from build123d import *

# Parameters (mm, degrees)
PAD_DEPTH    = 9
SKETCH001_R  = 2.5
POCKET_DEPTH = 10


with BuildPart() as part:
    # Sketch → Pad (new body)
    with BuildSketch(Plane.YZ):
        with BuildLine():
            Line((-3.5, 0), (-3.403323, 1.122173))
            ThreePointArc((-3.31749, 2.118482), (-3.858561, 1.663244), (-3.403323, 1.122173))
            Line((-3.31749, 2.118482), (-3.220813, 3.240655))
            ThreePointArc((-3.13498, 4.236964), (-3.676052, 3.781726), (-3.220813, 3.240655))
            Line((-3.13498, 4.236964), (-3.038304, 5.359137))
            ThreePointArc((-2.95247, 6.355446), (-3.493542, 5.900208), (-3.038304, 5.359137))
            Line((-2.95247, 6.355446), (-2.855794, 7.477619))
            ThreePointArc((-2.76996, 8.473929), (-3.311032, 8.01869), (-2.855794, 7.477619))
            Line((-2.76996, 8.473929), (-2.673284, 9.596101))
            ThreePointArc((-2.58745, 10.592411), (-3.128522, 10.137173), (-2.673284, 9.596101))
            Line((-2.58745, 10.592411), (-2.490774, 11.714583))
            ThreePointArc((2.490774, 11.714583), (0, 14), (-2.490774, 11.714583))
            Line((2.490774, 11.714583), (2.58745, 10.592411))
            ThreePointArc((2.673284, 9.596101), (3.128522, 10.137173), (2.58745, 10.592411))
            Line((2.673284, 9.596101), (2.76996, 8.473929))
            ThreePointArc((2.855794, 7.477619), (3.311032, 8.01869), (2.76996, 8.473929))
            Line((2.855794, 7.477619), (2.95247, 6.355446))
            ThreePointArc((3.038304, 5.359137), (3.493542, 5.900208), (2.95247, 6.355446))
            Line((3.038304, 5.359137), (3.13498, 4.236964))
            ThreePointArc((3.220813, 3.240655), (3.676052, 3.781726), (3.13498, 4.236964))
            Line((3.220813, 3.240655), (3.31749, 2.118482))
            ThreePointArc((3.403323, 1.122173), (3.858561, 1.663244), (3.31749, 2.118482))
            Line((3.403323, 1.122173), (3.5, 0))
            Line((-3.5, 0), (3.5, 0))
        make_face()
    extrude(amount=PAD_DEPTH)

    # Sketch001 → Pocket (cut)
    with BuildSketch(Plane.YX):
        with Locations((0, 4.5)):
            Circle(SKETCH001_R)
    extrude(amount=-POCKET_DEPTH, mode=Mode.SUBTRACT)


solid = part.part
The listing builds one solid part. Answer for the finished solid, in the listing's coordinates (mm). A direction names the side the tool comes from. Give positions to 0.01 mm unless a question says otherwise; leave off trailing zeros. Loops run counter-clockwise (first coordinate to the right, second up) from the corner with the lowest first, then second, coordinate; pieces in that order, holes last. Notation, with made-up numbers: (86.5, 89) - (97.5, 89) arc R12 ccw to (97.5, 105) - close; hole circle Ø11 at (11, 7). An arc over 180 degrees is marked (long way). Answer as a JSON object with one key per item and string values.
1. For a pull along Z with two mould halves and no side action, classify faces 1 (the flat face through (5, 0, 10)), 2 (the cylindrical face through (4.44, -3.31, 8.03)), 3 (the flat face through (9, 0, 7)) as pulls with the +Z half, pulls with the -Z half, needs draft (parallel to the pull), parting line crosses it, or undercut.
Determined:
{"face 1": "pulls with the -Z half", "face 2": "undercut", "face 3": "needs draft"}
2. For faces 4 (the flat face through (4.437, -3.452, 0.553)), 5 (the flat face through (4.44, -2.54, 11.15)), 6 (the cylindrical face through (7, 0, 5)), 7 (the flat face through (4.437, 3.086, 4.806)), determine the directions among +Z, -Z, +X, -X, +Y, -Y from which every point of the face is accessible in a straight line to the end or side of a thin tool.
Determined:
{"face 4": "+X, -X, -Y", "face 5": "+Z, +X, -X, -Y", "face 6": "-Z", "face 7": "+X, -X, +Y"}
3. A cutting plane is placed at D-D (x = 4.5). Write down the section's boundary in (y, z), then the cut area to 3 significant figures.
Determined:
{"outline": "(-3.5, 0) - (-2.5, 0) - (-2.5, 10) - (2.5, 10) - (2.5, 0) - (3.5, 0) - (3.4, 1.12) arc R0.5 ccw to (3.32, 2.12) - (3.22, 3.24) arc R0.5 ccw to (3.13, 4.24) - (3.04, 5.36) arc R0.5 ccw to (2.95, 6.36) - (2.86, 7.48) arc R0.5 ccw to (2.77, 8.47) - (2.67, 9.6) arc R0.5 ccw to (2.59, 10.59) - (2.49, 11.71) arc R2.5 ccw to (-2.49, 11.71) - (-2.59, 10.59) arc R0.5 ccw to (-2.67, 9.6) - (-2.77, 8.47) arc R0.5 ccw to (-2.86, 7.48) - (-2.95, 6.36) arc R0.5 ccw to (-3.04, 5.36) - (-3.13, 4.24) arc R0.5 ccw to (-3.22, 3.24) - (-3.32, 2.12) arc R0.5 ccw to (-3.4, 1.12) - close", "area": "32.9 mm²"}
4. A cutting plane is placed at B-B (x = 8.25). Write down the section's boundary in (y, z), then the cut area to 3 significant figures.
Determined:
{"outline": "(-3.5, 0) - (3.5, 0) - (3.4, 1.12) arc R0.5 ccw to (3.32, 2.12) - (3.22, 3.24) arc R0.5 ccw to (3.13, 4.24) - (3.04, 5.36) arc R0.5 ccw to (2.95, 6.36) - (2.86, 7.48) arc R0.5 ccw to (2.77, 8.47) - (2.67, 9.6) arc R0.5 ccw to (2.59, 10.59) - (2.49, 11.71) arc R2.5 ccw to (-2.49, 11.71) - (-2.59, 10.59) arc R0.5 ccw to (-2.67, 9.6) - (-2.77, 8.47) arc R0.5 ccw to (-2.86, 7.48) - (-2.95, 6.36) arc R0.5 ccw to (-3.04, 5.36) - (-3.13, 4.24) arc R0.5 ccw to (-3.22, 3.24) - (-3.32, 2.12) arc R0.5 ccw to (-3.4, 1.12) - close", "area": "82.9 mm²"}
5. Flat-ended cylindrical pins translate along their axes: pin 1 Ø3 at (x, y) = (4.5, 0) entering from -Z; pin 2 Ø1.5 at (x, z) = (4, 11) entering from -Y. Find the tip coordinate at first contact, or state that the pin passes through.
Determined:
{"pin 1": "z = 10", "pin 2": "y = -3.11"}
6. Find the intervals of material crossed by L1, parallel to X at y = 0, z = 6.75; L2, parallel to Z at x = 0.75, y = 3; L3, parallel to Z at x = 3, y = -0.5, in increasing order. Write a range as [from, to].
Determined:
{"L1": "[0, 2], [7, 9]", "L2": "[0, 6.36], [7.51, 8.44], [9.76, 10.43]", "L3": "[10, 13.95]"}
7. A cutting plane is placed at A-A (y = 0). Write down the section's boundary in (x, z), then the cut area to 3 significant figures.
Determined:
{"outline": "(0, 0) - (2, 0) - (2, 10) - (7, 10) - (7, 0) - (9, 0) - (9, 14) - (0, 14) - close", "area": "76.0 mm²"}
8. A cutting plane is placed at C-C (z = 7). Write down the section's boundary in (x, y), then the cut area to 3 significant figures.
Determined:
{"outline": "(0, -2.9) - (9, -2.9) - (9, 2.9) - (0, 2.9) - close; hole circle Ø5 at (4.5, 0)", "area": "32.5 mm²"}
